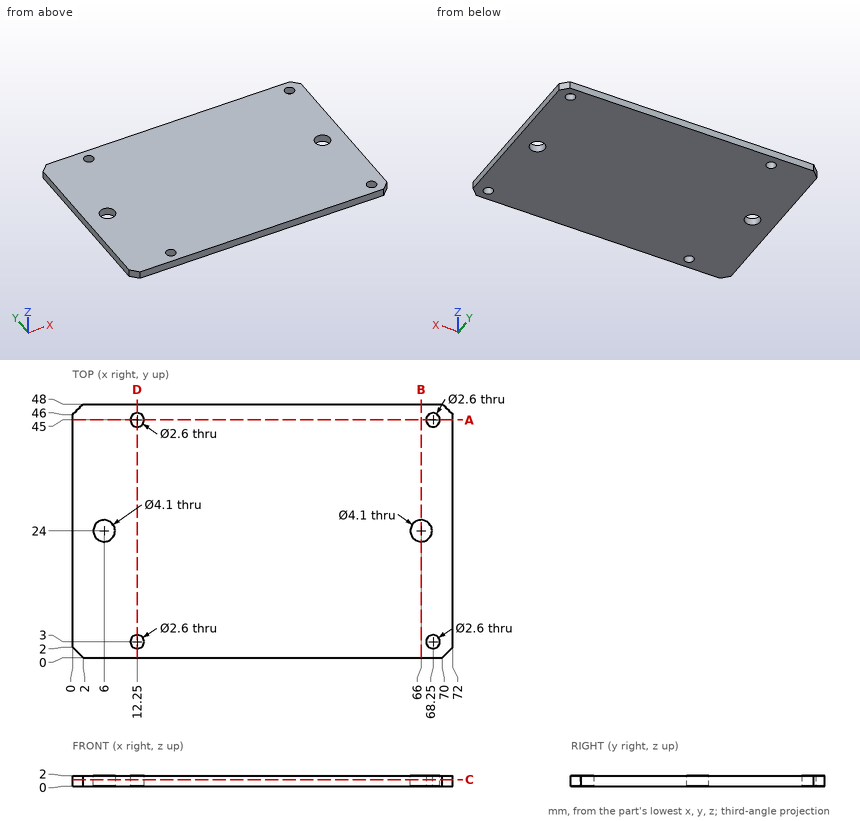
Answer from the drawing. Dimensions are ordinates in mm from the lowest x, y and z of the part. Give positions to 0.01 mm unless a question says otherwise; leave off trailing zeros. Loops run counter-clockwise (first coordinate to the right, second up) from the corner with the lowest first, then second, coordinate; pieces in that order, holes last. Notation, with made-up numbers: (-26, -10) - (-7, -10) arc R24 cw to (-7, 12) - close; hole circle Ø11 at (18, 52.5). An arc over 180 degrees is marked (long way). Write each question's results on one line, items separated by ' | '.
1. Find section C-C, the plane z = 1.25. Write down the section's boundary in (x, y).
Resolved:
outline: (0, 2) - (2, 0) - (70, 0) - (72, 2) - (72, 46) - (70, 48) - (2, 48) - (0, 46) - close; hole circle Ø4.1 at (6, 24); hole circle Ø2.6 at (12.25, 3); hole circle Ø2.6 at (12.25, 45); hole circle Ø4.1 at (66, 24); hole circle Ø2.6 at (68.25, 3); hole circle Ø2.6 at (68.25, 45)
2. Find section B-B, the plane x = 66. Write down the section's boundary in (y, z).
Resolved:
outline: (0, 0) - (21.95, 0) - (21.95, 2) - (0, 2) - close; (26.05, 0) - (48, 0) - (48, 2) - (26.05, 2) - close
3. Flat-ended cylindrical pins translate along their axes: P1, Ø3.5, axis at x = 6, y = 24, coming from the -Z side; P2, Ø5.5, axis at x = 66, y = 24, coming from the -Z side. Find the tip coordinate at first contact, or state that the pin passes through.
Resolved:
P1: passes through | P2: stops at z = 0
4. Find section A-A, the plane y = 45. Write down the section's boundary in (x, z), then the cut area to 3 significant figures.
Resolved:
outline: (0, 0) - (10.95, 0) - (10.95, 2) - (0, 2) - close; (13.55, 0) - (66.95, 0) - (66.95, 2) - (13.55, 2) - close; (69.55, 0) - (72, 0) - (72, 2) - (69.55, 2) - close | area: 134 mm^2
5. Consider probe 1 along Y at (x, z) = (68.25, 1); probe 2 along X at (y, z) = (45, 1.2); probe 3 along Y at (x, z) = (66, 0.6). Determine where each line is inside the solid, lowest interval first. Write a range as from..to.
Resolved:
probe 1: y = 0..1.7, 4.3..43.7, 46.3..48 | probe 2: x = 0..10.95, 13.55..66.95, 69.55..72 | probe 3: y = 0..21.95, 26.05..48
6. Find section D-D, the plane x = 12.25. Write down the section's boundary in (y, z).
Resolved:
outline: (0, 0) - (1.7, 0) - (1.7, 2) - (0, 2) - close; (4.3, 0) - (43.7, 0) - (43.7, 2) - (4.3, 2) - close; (46.3, 0) - (48, 0) - (48, 2) - (46.3, 2) - close
